Verification items for the finished model (mm, model axes). A direction names the side the tool comes from. Coordinates: 2 decimals unless noted, no trailing zeros. Order: outer loops, then holes, each group sorted by start corner. A loop starts at its lowest first (then second) coordinate and runs counter-clockwise, first axis right, second up. Notation, with made-up numbers: M -12.5,-34 L 24.5,-34 A22 ccw 24.5,-4 Z; hole C 27,17 d3. An arc over 180 degrees is marked long. Return JSON: item names as keys, results as strings. Group by question number.
1. Set-up check for faces 1 (the flat face through (-0.96, 12.17, -13.51)), 2 (the cylindrical face through (20, 18, -15)), 3 (the cylindrical face through (0.27, 4.86, -11.6)), 4 (the flat face through (-11.5, 2, 0)): record each of +Z, -Z, +X, -X, +Y, -Y from which the full face is reachable in a straight line by a thin tool's end or side.
2. Material ranges on line 1 along Z through (x, y) = (2, 18.5); line 2 along Y through (x, z) = (-2.5, -9); line 3 along Z through (x, y) = (-13.5, 5.25), recorded low to high.
3. Section check D-D, the plane x = 2. Record the cut outline in (y, z).
4. Section check C-C, the plane z = 0.5. Record the cut outline in (x, y), plus the area to 3 significant figures.
5. Section check B-B, the plane y = 5.75. Record the cut outline in (x, z).
6. Gauge pin test, flat ends, axial feed: pin 1 (3 mm diameter, centred on x = 5.5, y = 1.5, fed in from -Z); pin 2 (1.8 mm diameter, centred on x = 0, y = 1, fed in from +Z); pin 3 (1.2 mm diameter, centred on y = 1.5, z = 2.5, fed in from +X); pin 4 (8 mm diameter, centred on y = 9.5, z = -4, fed in from +X). Record the tip position at first contact, or that the pin passes through.
7. Section check A-A, the plane x = 12. Record the cut outline in (y, z), plus the area to 3 significant figures.
8. Mould release check, pull along Z, two halves, no side actions. Record for faces 5 (the flat face through (-0.96, 12.17, 13.49)), 6 (the flat face through (0, 1, -11)), 7 (the flat face through (0, 2, -6.15)): +Z half, -Z half, draft (parallel to the pull), parting line (faces both ways), or undercut.
```python
from build123d import *

# Parameters (mm, degrees)
SKETCH1_W           = 38
SKETCH1_H           = 22
SKETCH1_W_2         = 23
SKETCH1_H_2         = 12.3
BOSS_EXTRUDE1_DEPTH = 4
BOSS_EXTRUDE2_DEPTH = 42
FILLET1_R           = 3
SKETCH4_W           = 4
SKETCH4_H           = 4.046186486
CUT_EXTRUDE1_DEPTH  = 44.058100283
CUT_EXTRUDE2_DEPTH  = 44.058100283
SKETCH7_R           = 1
BOSS_EXTRUDE3_DEPTH = 1.2
FILLET2_R           = 0.5


with BuildPart() as part:
    # Sketch1 → Boss-Extrude1 (new body)
    with BuildSketch(Plane(origin=(0, 0, 0), x_dir=(1, 0, 0), z_dir=(0, 1, 0))):
        Rectangle(SKETCH1_W, SKETCH1_H)
        Rectangle(SKETCH1_W_2, SKETCH1_H_2, mode=Mode.SUBTRACT)
    extrude(amount=BOSS_EXTRUDE1_DEPTH)

    # Sketch2 → Boss-Extrude2 (add)
    with BuildSketch(Plane.ZY.offset(19)):
        Polygon((-11, 2.2), (-14.5, 2.2), (-14.5, 22), (-12.5, 22), (-12.5, 4), (-11, 4), align=None)
        Polygon((12.5, 4), (11, 4), (11, 2.2), (14.5, 2.2), (14.5, 22), (12.5, 22), align=None)
    extrude(amount=-BOSS_EXTRUDE2_DEPTH)

    # Fillet1
    fillet1_edges = [part.edges().sort_by_distance(p)[0] for p in [
        (2, 2.2, 14.5),
        (2, 2.2, -14.5),
        (2, 4, 12.5),
        (2, 4, -12.5),
    ]]
    fillet(fillet1_edges, radius=FILLET1_R)

    # Sketch4 → Cut-Extrude1 (cut, through all)
    with BuildSketch(Plane(origin=(0, 0, -14.5), x_dir=(-1, 0, 0), z_dir=(0, 0, -1))):
        with Locations((-21, 3.176906757)):
            Rectangle(SKETCH4_W, SKETCH4_H)
        with BuildLine():
            Line((-23, 5.2), (-19, 5.2))
            Line((-19, 5.2), (-19, 16))
            Line((-19, 16), (-20, 16))
            ThreePointArc((-20, 16), (-22.121320344, 16.878679656), (-23, 19))
            Line((-23, 19), (-23, 5.2))
        make_face()
        with BuildLine():
            ThreePointArc((-23, 19), (-22.121320344, 21.121320344), (-20, 22))
            Line((-20, 22), (-23, 22))
            Line((-23, 22), (-23, 19))
        make_face()
        Polygon((-0.991025267, 22), (17.667264982, 5.2), (19, 5.2), (19, 22), align=None)
        Polygon((17.667264982, 5.2), (19, 4), (19, 5.2), align=None)
    extrude(amount=-CUT_EXTRUDE1_DEPTH, mode=Mode.SUBTRACT)

    # Sketch6 → Cut-Extrude2 (cut, through all)
    with BuildSketch(Plane(origin=(0, 0, -14.5), x_dir=(-1, 0, 0), z_dir=(0, 0, -1))):
        Polygon((6.479180653, 7.2), (-13, 7.2), (-13, 17), (-4.404821992, 17), align=None)
    extrude(amount=-CUT_EXTRUDE2_DEPTH, mode=Mode.SUBTRACT)

    # Sketch7 → Boss-Extrude3 (add)
    with BuildSketch(Plane(origin=(0, 0, -14.5), x_dir=(-1, 0, 0), z_dir=(0, 0, -1))):
        with Locations((-20, 19)):
            Circle(SKETCH7_R)
    extrude(amount=BOSS_EXTRUDE3_DEPTH)

    # Fillet2
    fillet2_edges = [part.edges().sort_by_distance(p)[0] for p in [
        (21, 19, -15.7),
    ]]
    fillet(fillet2_edges, radius=FILLET2_R)


solid = part.part
```
Answers follow:
{
 "1": {"face 1": "+Z, -Z", "face 2": "-Z", "face 3": "+X, -X, +Y", "face 4": "+Y, -Y"},
 "2": {"line 1": "-14.5 to -12.5, 12.5 to 14.5", "line 2": "0 to 4", "line 3": "-14.5 to -11.94, 11.94 to 14.5"},
 "3": {"outline": "M 0,-11 L 2.2,-11 L 2.2,-11.5 A3 ccw 5.2,-14.5 L 7.2,-14.5 L 7.2,-12.5 L 7,-12.5 A3 cw 4,-9.5 L 4,-6.15 L 0,-6.15 Z; M 0,6.15 L 4,6.15 L 4,9.5 A3 cw 7,12.5 L 7.2,12.5 L 7.2,14.5 L 5.2,14.5 A3 ccw 2.2,11.5 L 2.2,11 L 0,11 Z; M 14.83,-14.5 L 22,-14.5 L 22,-12.5 L 14.83,-12.5 Z; M 14.83,12.5 L 22,12.5 L 22,14.5 L 14.83,14.5 Z"},
 "4": {"outline": "M -19,0 L -11.5,0 L -11.5,4 L -19,4 Z; M 11.5,0 L 19,0 L 19,4 L 11.5,4 Z", "area": "60.0 mm^2"},
 "5": {"outline": "M -17.06,-14.5 L 19,-14.5 L 19,-12.23 L -17.06,-12.23 Z; M -17.06,12.23 L 19,12.23 L 19,14.5 L -17.06,14.5 Z"},
 "6": {"pin 1": "z = -13.54", "pin 2": "z = 11", "pin 3": "x = 19", "pin 4": "through"},
 "7": {"outline": "M 0,-11 L 2.2,-11 L 2.2,-11.5 A3 ccw 5.2,-14.5 L 7.2,-14.5 L 7.2,-12.5 L 7,-12.5 A3 cw 4,-9.5 L 4,9.5 A3 cw 7,12.5 L 7.2,12.5 L 7.2,14.5 L 5.2,14.5 A3 ccw 2.2,11.5 L 2.2,11 L 0,11 Z; M 17,-14.5 L 22,-14.5 L 22,-12.5 L 17,-12.5 Z; M 17,12.5 L 22,12.5 L 22,14.5 L 17,14.5 Z", "area": "133 mm^2"},
 "8": {"face 5": "draft", "face 6": "-Z half", "face 7": "undercut"}
}
